Check sheet for the modelled part. Datum: model origin and axes. Units: mm. Round coordinates to 2 decimals unless told otherwise and drop trailing zeros. Write each loop counter-clockwise with the first axis right and the second up, starting at its lowest first coordinate (ties: lowest second). Pieces come first, ordered by that corner, then holes.
Item 1: Depth check by flat-ended pin: pin 1 (0.9 mm diameter, centred on x = -29.5, y = -0.5, fed in from +Z). Enter the tip coordinate at first touch or a pass-through.
Item 2: Material ranges on line 1 along X through (y, z) = (-1.05, 12.25); line 2 along X through (y, z) = (0.75, 23.5), recorded low to high.
Item 3: Section check B-B, the plane z = 24.5. Record the cut outline in (x, y), plus the area to 3 significant figures.
Item 4: Section check A-A, the plane y = -0.25. Record the cut outline in (x, z).
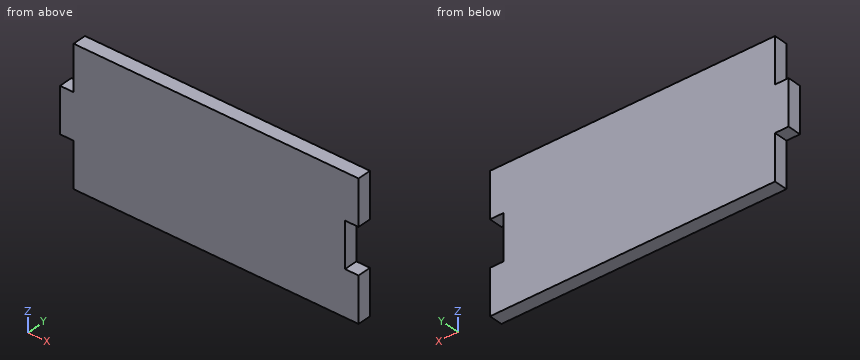
from build123d import *

# Parameters (mm, degrees)
F0_W     = 60
F0_H     = 3
F1_DEPTH = 30
F2_W     = 3
F2_H     = 10
F3_DEPTH = 3
F4_W     = 3
F4_H     = 10
F5_DEPTH = 3


with BuildPart() as f1:
    # F0 (on Top) → F1 (new body)
    with BuildSketch(Plane.XY):
        with Locations((1.74342, -0.519499)):
            Rectangle(F0_W, F0_H)
    extrude(amount=F1_DEPTH)

    # F2 (on face) → F3 (join)
    with BuildSketch(Plane.YZ.offset(31.74342)):
        with Locations((-0.519499, 25)):
            Rectangle(F2_W, F2_H)
        with Locations((-0.519499, 5)):
            Rectangle(F2_W, F2_H)
    extrude(amount=F3_DEPTH)

    # F4 (on face) → F5 (join)
    with BuildSketch(Plane(origin=(-28.25658, 0, 0), x_dir=(0, -1, 0), z_dir=(-1, 0, 0))):
        with Locations((0.519499, 15)):
            Rectangle(F4_W, F4_H)
    extrude(amount=F5_DEPTH)


solid = f1.part
Values found:
1. pin 1: stops at z = 20
2. line 1: x = -31.26 to 31.74
2. line 2: x = -28.26 to 34.74
3. outline: (-28.26, -2.02) - (34.74, -2.02) - (34.74, 0.98) - (-28.26, 0.98) - close
3. area: 189 mm2
4. outline: (-31.26, 10) - (-28.26, 10) - (-28.26, 0) - (34.74, 0) - (34.74, 10) - (31.74, 10) - (31.74, 20) - (34.74, 20) - (34.74, 30) - (-28.26, 30) - (-28.26, 20) - (-31.26, 20) - close
